Check sheet for the drawn part. Datum: minimum x, y, z corner. Units: mm. A direction names the side the tool comes from. Round coordinates to 2 decimals unless told otherwise and drop trailing zeros. Order: outer loops, then holes, each group sorted by start corner. A loop starts at its lowest first (then second) coordinate and runs counter-clockwise, first axis right, second up.
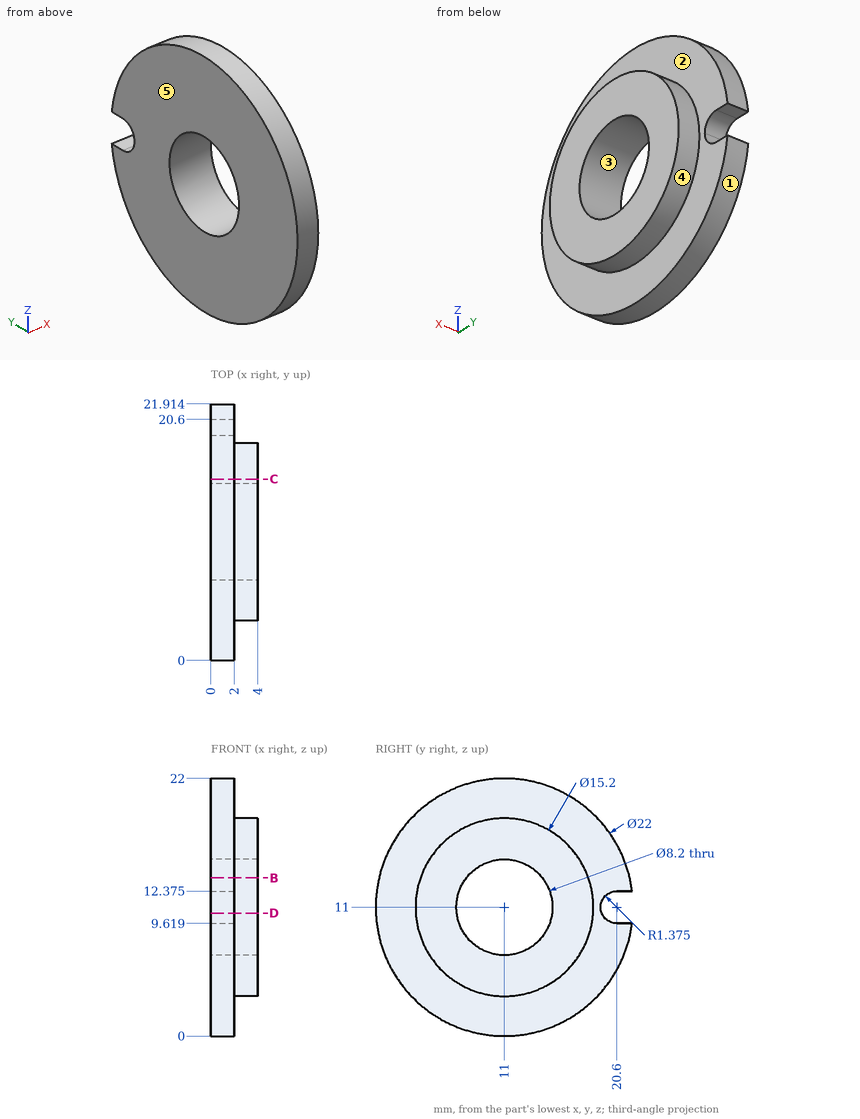
(1) Depth check by flat-ended pin: P1, Ø1.4, axis at x = 1.5, y = 21, coming from the +Z side (1 decimal); P2, Ø5, axis at y = 11, z = 11, coming from the -X side; P3, Ø1.5, axis at y = 18.5, z = 13.5, coming from the -X side; P4, Ø2, axis at x = 2, y = 6.5, coming from the +Z side. Enter the tip coordinate at first touch or a pass-through.
Returned:
P1: stops at z = 16.9
P2: passes through
P3: stops at x = 0
P4: stops at z = 21.43
(2) Draft check along Z on the marked faces 1, 2 and 3. Enter one of: released by +Z, released by -Z, zero draft, split by the parting line, or undercut.
Returned:
face 1: split by the parting line
face 2: zero draft
face 3: undercut
(3) Sectioned sample at B-B, the plane z = 13.5. Record the cut outline in (x, y).
Returned:
outline: (0, 0.29) - (2, 0.29) - (2, 3.82) - (4, 3.82) - (4, 7.75) - (0, 7.75) - close; (0, 14.25) - (4, 14.25) - (4, 18.18) - (2, 18.18) - (2, 21.71) - (0, 21.71) - close
(4) Set-up check for the marked faces 4 and 5: record each of +Z, -Z, +X, -X, +Y, -Y from which the full face is reachable in a straight line by a thin tool's end or side.
Returned:
face 4: +X
face 5: +Z, -Z, -X, +Y, -Y
(5) Sectioned sample at D-D, the plane z = 10.5. Record the cut outline in (x, y).
Returned:
outline: (0, 0.01) - (2, 0.01) - (2, 3.42) - (4, 3.42) - (4, 6.93) - (0, 6.93) - close; (0, 15.07) - (4, 15.07) - (4, 18.58) - (2, 18.58) - (2, 19.32) - (0, 19.32) - close
(6) Material ranges on line 1 (Z direction, x = 3.25, y = 11); line 2 (Z direction, x = 1.4, y = 11); line 3 (X direction, y = 4.5, z = 4.75), recorded low to high.
Returned:
line 1: z = 3.4 to 6.9, 15.1 to 18.6
line 2: z = 0 to 6.9, 15.1 to 22
line 3: x = 0 to 2
(7) Sectioned sample at C-C, the plane y = 15.5. Record the cut outline in (x, z) (1 decimal).
Returned:
outline: (0, 1) - (2, 1) - (2, 4.9) - (4, 4.9) - (4, 17.1) - (2, 17.1) - (2, 21) - (0, 21) - close
